Can you work these out from the drawing? Everything is in mm from the part's minimum corner. Coordinates: 2 decimals unless noted, no trailing zeros. Loops run counter-clockwise (first coordinate to the right, second up) from the corner with the lowest first, then second, coordinate; pieces in that order, holes last. Notation, with made-up numbers: M 7.25,19 L 66.25,19 A23 ccw 66.25,40 Z; hole C -4,-13.5 d5. An arc over 180 degrees is marked long. Write each question's results on one line, items separated by ' | '.
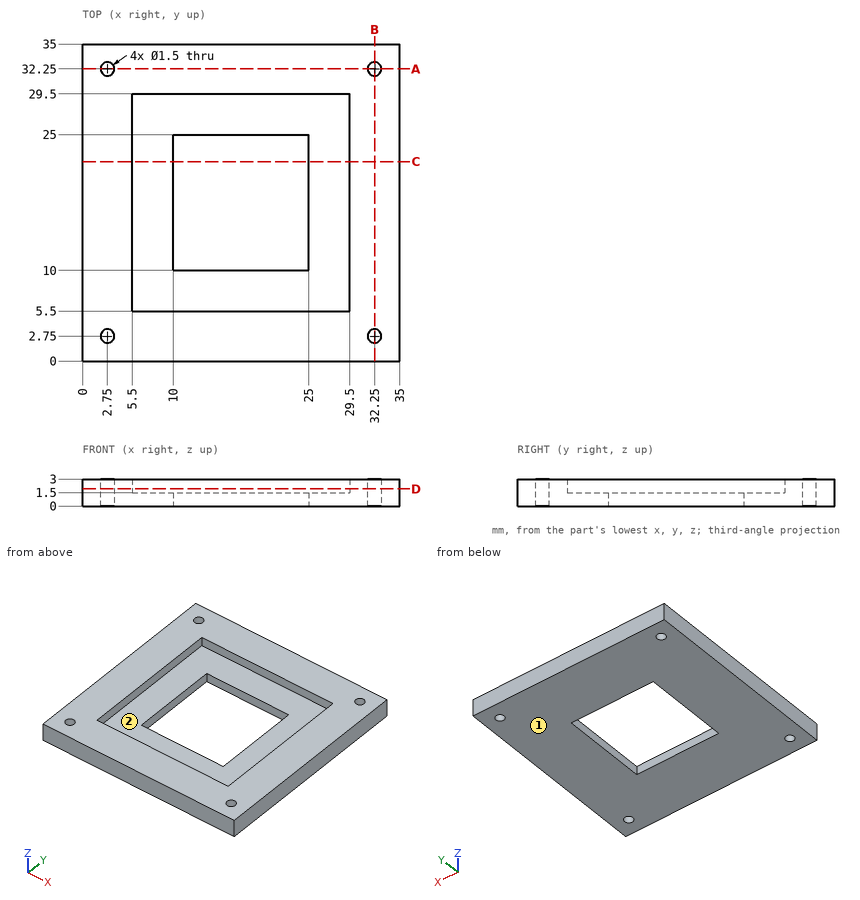
(1) Imagine slicing it at C-C, the plane y = 22. List the corners of the cut face in (x, z) for me, and give its area (3 significant figures).
Reported:
outline: M 0,0 L 10,0 L 10,1.5 L 5.5,1.5 L 5.5,3 L 0,3 Z; M 25,0 L 35,0 L 35,3 L 29.5,3 L 29.5,1.5 L 25,1.5 Z | area: 46.5 mm2
(2) Will these pins go through, and if not, where does the flat tip stop? P1, Ø12, axis at x = 15.5, y = 12, coming from the +Z side; P2, Ø1.7, axis at x = 32.25, y = 2.75, coming from the +Z side.
Reported:
P1: stops at z = 1.5 | P2: stops at z = 3
(3) If we mould it in two halves opening along X, with no side actions, what happens to the marked faces 1 and 2? For each: released by +X, released by -X, zero draft, split by the parting line, or undercut.
Reported:
face 1: zero draft | face 2: undercut
(4) Imagine slicing it at A-A, the plane y = 32.25. List the corners of the cut face in (x, z) for me.
Reported:
outline: M 0,0 L 2,0 L 2,3 L 0,3 Z; M 3.5,0 L 31.5,0 L 31.5,3 L 3.5,3 Z; M 33,0 L 35,0 L 35,3 L 33,3 Z
(5) Imagine slicing it at D-D, the plane z = 1.9. List the corners of the cut face in (x, y) for me, and give its area (3 significant figures).
Reported:
outline: M 0,0 L 35,0 L 35,35 L 0,35 Z; hole C 2.75,2.75 d1.5; hole C 2.75,32.25 d1.5; hole M 5.5,5.5 L 29.5,5.5 L 29.5,29.5 L 5.5,29.5 Z; hole C 32.25,2.75 d1.5; hole C 32.25,32.25 d1.5 | area: 642 mm2
(6) Please list where these lines run through material, in increasing order: probe 1 along Y at (x, z) = (32.25, 1.75); probe 2 along Y at (x, z) = (24, 0.9). Write a range as from..to.
Reported:
probe 1: y = 0..2, 3.5..31.5, 33..35 | probe 2: y = 0..10, 25..35
